For this review, take the finished solid that the model builds, in its own axes (mm). Round coordinates to 2 decimals unless told otherwise and drop trailing zeros. Write each loop counter-clockwise with the first axis right and the second up, starting at its lowest first coordinate (ties: lowest second). Pieces come first, ordered by that corner, then holes. Notation, with made-up numbers: (31, -17.75) -> (69, -17.75) arc R16 cw to (69, 11.25) -> close; hole circle Ø6 at (44, 52). An arc over 180 degrees is marked (long way). Write item = value, one per line. Start each with the question number.
```python
from build123d import *

# Parameters (mm, degrees)
BASE_FLANGE1_DEPTH  = 4.5
CUT_EXTRUDE1_DEPTH  = 235.407023146
SKETCH7_W           = 25.2
SKETCH7_H           = 2.55
CUT_EXTRUDE2_DEPTH  = 10
SKETCH8_W           = 3
SKETCH8_H           = 25
BOSS_EXTRUDE1_DEPTH = 4.5
CUT_EXTRUDE3_START  = -4.55
SKETCH10_W          = 0.35
SKETCH10_H          = 23.55
SKETCH10_H_2        = 20
CUT_EXTRUDE3_DEPTH  = 4.55
SKETCH11_R          = 2.65
CUT_EXTRUDE4_DEPTH  = 238.093473128


# Sheet-metal steps are written as plain solids
with BuildPart() as part:
    # Sketch1 → Base-Flange1 (new body)
    with BuildSketch(Plane(origin=(0, 0, 0), x_dir=(1, 0, 0), z_dir=(0, 1, 0))):
        with BuildLine():
            Line((-219.25, 79.3), (219.25, 79.3))
            Line((219.25, 79.3), (219.25, -79.3))
            ThreePointArc((219.25, -79.3), (218.224873734, -81.774873734), (215.75, -82.8))
            Line((215.75, -82.8), (-215.75, -82.8))
            ThreePointArc((-215.75, -82.8), (-218.224873734, -81.774873734), (-219.25, -79.3))
            Line((-219.25, -79.3), (-219.25, 79.3))
        make_face()
    extrude(amount=-BASE_FLANGE1_DEPTH)

    # Sketch6 → Cut-Extrude1 (cut, through all)
    with BuildSketch(Plane(origin=(0, 0, 0), x_dir=(1, 0, 0), z_dir=(0, 1, 0))):
        with BuildLine():
            Line((-198.45, 60.25), (-85.25, 60.25))
            ThreePointArc((-85.25, 60.25), (-84.012563133, 59.737436867), (-83.5, 58.5))
            Line((-83.5, 58.5), (-83.5, -62))
            ThreePointArc((-83.5, -62), (-84.012563133, -63.237436867), (-85.25, -63.75))
            Line((-85.25, -63.75), (-198.45, -63.75))
            ThreePointArc((-198.45, -63.75), (-199.687436867, -63.237436867), (-200.2, -62))
            Line((-200.2, -62), (-200.2, 58.5))
            ThreePointArc((-200.2, 58.5), (-199.687436867, 59.737436867), (-198.45, 60.25))
        make_face()
        with BuildLine():
            Line((200.2, 58.5), (200.2, -62))
            ThreePointArc((200.2, -62), (199.687436867, -63.237436867), (198.45, -63.75))
            Line((198.45, -63.75), (85.25, -63.75))
            ThreePointArc((85.25, -63.75), (84.012563133, -63.237436867), (83.5, -62))
            Line((83.5, -62), (83.5, 58.5))
            ThreePointArc((83.5, 58.5), (84.012563133, 59.737436867), (85.25, 60.25))
            Line((85.25, 60.25), (198.45, 60.25))
            ThreePointArc((198.45, 60.25), (199.687436867, 59.737436867), (200.2, 58.5))
        make_face()
        with BuildLine():
            Line((63.5, 58.5), (63.5, -62))
            ThreePointArc((63.5, -62), (62.987436867, -63.237436867), (61.75, -63.75))
            Line((61.75, -63.75), (-61.75, -63.75))
            ThreePointArc((-61.75, -63.75), (-62.987436867, -63.237436867), (-63.5, -62))
            Line((-63.5, -62), (-63.5, 58.5))
            ThreePointArc((-63.5, 58.5), (-62.987436867, 59.737436867), (-61.75, 60.25))
            Line((-61.75, 60.25), (61.75, 60.25))
            ThreePointArc((61.75, 60.25), (62.987436867, 59.737436867), (63.5, 58.5))
        make_face()
    extrude(amount=-CUT_EXTRUDE1_DEPTH, mode=Mode.SUBTRACT)

    # Sketch7 → Cut-Extrude2 (cut)
    with BuildSketch(Plane(origin=(0, 0, 0), x_dir=(1, 0, 0), z_dir=(0, 1, 0))):
        with Locations((-186.75, 78.025)):
            Rectangle(SKETCH7_W, SKETCH7_H)
        with Locations((-93.375, 78.025)):
            Rectangle(SKETCH7_W, SKETCH7_H)
        with Locations((0, 78.025)):
            Rectangle(SKETCH7_W, SKETCH7_H)
        with Locations((93.375, 78.025)):
            Rectangle(SKETCH7_W, SKETCH7_H)
        with Locations((186.75, 78.025)):
            Rectangle(SKETCH7_W, SKETCH7_H)
    extrude(amount=-CUT_EXTRUDE2_DEPTH, mode=Mode.SUBTRACT)

    # Sketch8 → Boss-Extrude1 (add)
    with BuildSketch(Plane(origin=(0, 0, 0), x_dir=(1, 0, 0), z_dir=(0, 1, 0))):
        with Locations((220.75, -1.75)):
            Rectangle(SKETCH8_W, SKETCH8_H)
        with Locations((220.75, 46.8)):
            Rectangle(SKETCH8_W, SKETCH8_H)
        with Locations((220.75, -50.3)):
            Rectangle(SKETCH8_W, SKETCH8_H)
    boss_extrude1 = extrude(amount=-BOSS_EXTRUDE1_DEPTH)

    # Mirror1: Boss-Extrude1 across plane
    add(boss_extrude1.mirror(Plane(origin=(0, 0, 0), x_dir=(0, 0, 1), z_dir=(1, 0, 0))))

    # Sketch10 → Cut-Extrude3 (cut)
    with BuildSketch(Plane.XZ.offset(4.5).offset(CUT_EXTRUDE3_START)):
        with Locations((-219.075, 26.025)):
            Rectangle(SKETCH10_W, SKETCH10_H)
        with Locations((-219.075, -22.525)):
            Rectangle(SKETCH10_W, SKETCH10_H)
        with Locations((-219.075, -69.3)):
            Rectangle(SKETCH10_W, SKETCH10_H_2)
        with BuildLine():
            Line((218.9, 79.3), (218.9, 62.8))
            Line((218.9, 62.8), (219.25, 62.8))
            Line((219.25, 62.8), (219.25, 79.3))
            ThreePointArc((219.25, 79.3), (218.224873734, 81.774873734), (215.75, 82.8))
            Line((215.75, 82.8), (-215.75, 82.8))
            ThreePointArc((-215.75, 82.8), (-218.224873734, 81.774873734), (-219.25, 79.3))
            Line((-219.25, 79.3), (-219.25, 62.8))
            Line((-219.25, 62.8), (-218.9, 62.8))
            Line((-218.9, 62.8), (-218.9, 79.3))
            ThreePointArc((-218.9, 79.3), (-217.977386361, 81.527386361), (-215.75, 82.45))
            Line((-215.75, 82.45), (215.75, 82.45))
            ThreePointArc((215.75, 82.45), (217.977386361, 81.527386361), (218.9, 79.3))
        make_face()
        with Locations((219.075, 26.025)):
            Rectangle(SKETCH10_W, SKETCH10_H)
        with Locations((219.075, -22.525)):
            Rectangle(SKETCH10_W, SKETCH10_H)
        with Locations((219.075, -69.3)):
            Rectangle(SKETCH10_W, SKETCH10_H_2)
    extrude(amount=CUT_EXTRUDE3_DEPTH, mode=Mode.SUBTRACT)

    # Sketch11 → Cut-Extrude4 (cut, through all)
    with BuildSketch(Plane(origin=(0, 0, 0), x_dir=(1, 0, 0), z_dir=(0, 1, 0))):
        with Locations(Location((73.5, 47.8, 0), (0, 0, 270))):
            Circle(SKETCH11_R)
        with Locations(Location((73.5, 6.434271247, 0), (0, 0, 270))):
            Circle(SKETCH11_R)
        with Locations(Location((-73.5, 6.434271247, 0), (0, 0, 270))):
            Circle(SKETCH11_R)
        with Locations(Location((-73.5, 47.8, 0), (0, 0, 270))):
            Circle(SKETCH11_R)
    extrude(amount=-CUT_EXTRUDE4_DEPTH, mode=Mode.SUBTRACT)


solid = part.part
```
1. Consider section C-C, the plane z = 30. Give the boundary of the cut face in (x, y), then the cut area to 3 significant figures.
2. Consider section D-D, the plane x = -35. Give the boundary of the cut face in (y, z).
3. Consider section B-B, the plane x = -184. Give the boundary of the cut face in (y, z).
4. Consider section A-A, the plane z = 8.5. Give the boundary of the cut face in (x, y).
5. Wall thickness on L1, parallel to X at y = -3.5, z = 0.5; L2, parallel to X at y = -1.45, z = -47.8; L3, parallel to X at y = -0.9, z = -17: over which ranges is each line inside the solid? List them lowest first. Write a range as from..to.
6. Clearance check with flat-ended pins moving along their axes: pin 1 Ø2 at (y, z) = (-3, -67) entering from +X; pin 2 Ø2.5 at (x, y) = (-220.5, -3) entering from +Z; pin 3 Ø2 at (x, y) = (-3.5, -2.5) entering from -Z. State where each tip first meets the part, or that it passes through.
Outcome:
q1.outline = (-218.9, -4.5) -> (-200.2, -4.5) -> (-200.2, 0) -> (-218.9, 0) -> close; (-83.5, -4.5) -> (-63.5, -4.5) -> (-63.5, 0) -> (-83.5, 0) -> close; (63.5, -4.5) -> (83.5, -4.5) -> (83.5, 0) -> (63.5, 0) -> close; (200.2, -4.5) -> (218.9, -4.5) -> (218.9, 0) -> (200.2, 0) -> close
q1.area = 348 mm2
q2.outline = (-4.5, -79.3) -> (0, -79.3) -> (0, -60.25) -> (-4.5, -60.25) -> close; (-4.5, 63.75) -> (0, 63.75) -> (0, 82.45) -> (-4.5, 82.45) -> close
q3.outline = (-4.5, -76.75) -> (0, -76.75) -> (0, -60.25) -> (-4.5, -60.25) -> close; (-4.5, 63.75) -> (0, 63.75) -> (0, 82.45) -> (-4.5, 82.45) -> close
q4.outline = (-222.25, -4.5) -> (-200.2, -4.5) -> (-200.2, 0) -> (-222.25, 0) -> close; (-83.5, -4.5) -> (-63.5, -4.5) -> (-63.5, 0) -> (-83.5, 0) -> close; (63.5, -4.5) -> (83.5, -4.5) -> (83.5, 0) -> (63.5, 0) -> close; (200.2, -4.5) -> (222.25, -4.5) -> (222.25, 0) -> (200.2, 0) -> close
q5.L1 = -222.25..-200.2, -83.5..-63.5, 63.5..83.5, 200.2..222.25
q5.L2 = -222.25..-200.2, -83.5..-76.15, -70.85..-63.5, 63.5..70.85, 76.15..83.5, 200.2..222.25
q5.L3 = -218.9..-200.2, -83.5..-63.5, 63.5..83.5, 200.2..218.9
q6.pin_1 = 218.9
q6.pin_2 = 62.8
q6.pin_3 = -76.75
